Source: CAD feature listing. Evaluate the final solid. Frame: model axes, mm. A direction names the side the tool comes from. Coordinates: 2 decimals unless noted, no trailing zeros. Order: outer loops, then holes, each group sorted by start corner. A loop starts at its lowest first (then second) coordinate and runs counter-clockwise, first axis right, second up. Notation, with made-up numbers: (-18, -3.5) - (37, -3.5) arc R15 ccw to (37, 7.5) - close; hole circle Ø1 at (64, -24.75). An arc over 180 degrees is marked (long way). One line per question, with ' | ' between items. Start each with the question number.
(1) Access query for faces 1 (the flat face through (-165, 0, 312)), 2 (the flat face through (-3, 1, 320)). Directions: +Z, -Z, +X, -X, +Y, -Y. A direction counts if a zero-diameter tool reaches every point of the face in a straight line with its end or side. Return the directions, or none.
(2) Section B-B (x = -157.5). Return the cut outline in (y, z).
(3) Section A-A (y = -50). Return the cut outline in (x, z) (3 decimals).
(4) Draft query along X for faces 3 (the flat face through (-200, -1, 312)), 4 (the flat face through (-3, -100, 312)), 5 (the flat face through (-95, 0, 312)), 6 (the flat face through (-58, -65, 312)). Return one class per face: +X half, -X half, draft (parallel to the pull), parting line (faces both ways), or undercut.
(5) Section C-C (z = 309.25). Return the cut outline in (x, y) (3 decimals), then the cut area to 3 significant figures.
(6) Line query: line 1 along X through (y, z) = (21, 308) (3 decimals); line 2 along X through (y, z) = (-37, 310) (3 decimals); line 3 along Y through (x, z) = (-120.5, 312). Output: solid intervals per line, ascending.
from build123d import *

# Parameters (mm, degrees)
SKETCH053_W     = 400
SKETCH053_H     = 200
PAD027_DEPTH    = 15
SKETCH052_W     = 70
SKETCH052_H     = 60
POCKET018_DEPTH = 15
SKETCH061_W     = 21
SKETCH061_H     = 130
POCKET020_DEPTH = 15.001


with BuildPart() as part:
    # Sketch053 → Pad027 (new body)
    with BuildSketch(Plane.XY):
        Rectangle(SKETCH053_W, SKETCH053_H)
    extrude(amount=PAD027_DEPTH)

    # Sketch052 → Pocket018 (cut)
    with BuildSketch(Plane.XY):
        with Locations((-130, 0)):
            Rectangle(SKETCH052_W, SKETCH052_H)
    extrude(amount=POCKET018_DEPTH, mode=Mode.SUBTRACT)

    # Sketch061 → Pocket020 (cut, through all)
    with BuildSketch(Plane.XY):
        with Locations((-57.925, 0)):
            Rectangle(SKETCH061_W, SKETCH061_H)
    extrude(amount=POCKET020_DEPTH, mode=Mode.SUBTRACT)


with BuildPart() as part_1:
    # Body052 placement: moved
    add(part.part.moved(Location((0, 0, 305))))


solid = part_1.part
Response values:
1) face 1: +Z, -Z | face 2: +Z, +X, -X, +Y, -Y
2) outline: (-100, 305) - (-30, 305) - (-30, 320) - (-100, 320) - close; (30, 305) - (100, 305) - (100, 320) - (30, 320) - close
3) outline: (-200, 305) - (-68.425, 305) - (-68.425, 320) - (-200, 320) - close; (-47.425, 305) - (200, 305) - (200, 320) - (-47.425, 320) - close
4) face 3: -X half | face 4: draft | face 5: undercut | face 6: undercut
5) outline: (-200, -100) - (200, -100) - (200, 100) - (-200, 100) - close; hole (-165, -30) - (-95, -30) - (-95, 30) - (-165, 30) - close; hole (-68.425, -65) - (-47.425, -65) - (-47.425, 65) - (-68.425, 65) - close | area: 73,100 mm²
6) line 1: x = -200 to -165, -95 to -68.425, -47.425 to 200 | line 2: x = -200 to -68.425, -47.425 to 200 | line 3: y = -100 to -30, 30 to 100
